Could you check a few things on this drawing? It's one solid part, dimensions in mm from its lowest x, y, z. Give positions to 0.01 mm unless a question says otherwise; leave off trailing zeros. Order: outer loops, then holes, each group sorted by start corner. A loop starts at its lowest first (then second) coordinate and runs counter-clockwise, first axis right, second up. Notation, with made-up numbers: M -14.5,83.25 L 12.5,83.25 A23 ccw 12.5,117.25 Z; hole C 74.25,79.5 d1. An arc over 180 degrees is marked long. Use one line per item in the form item = value.
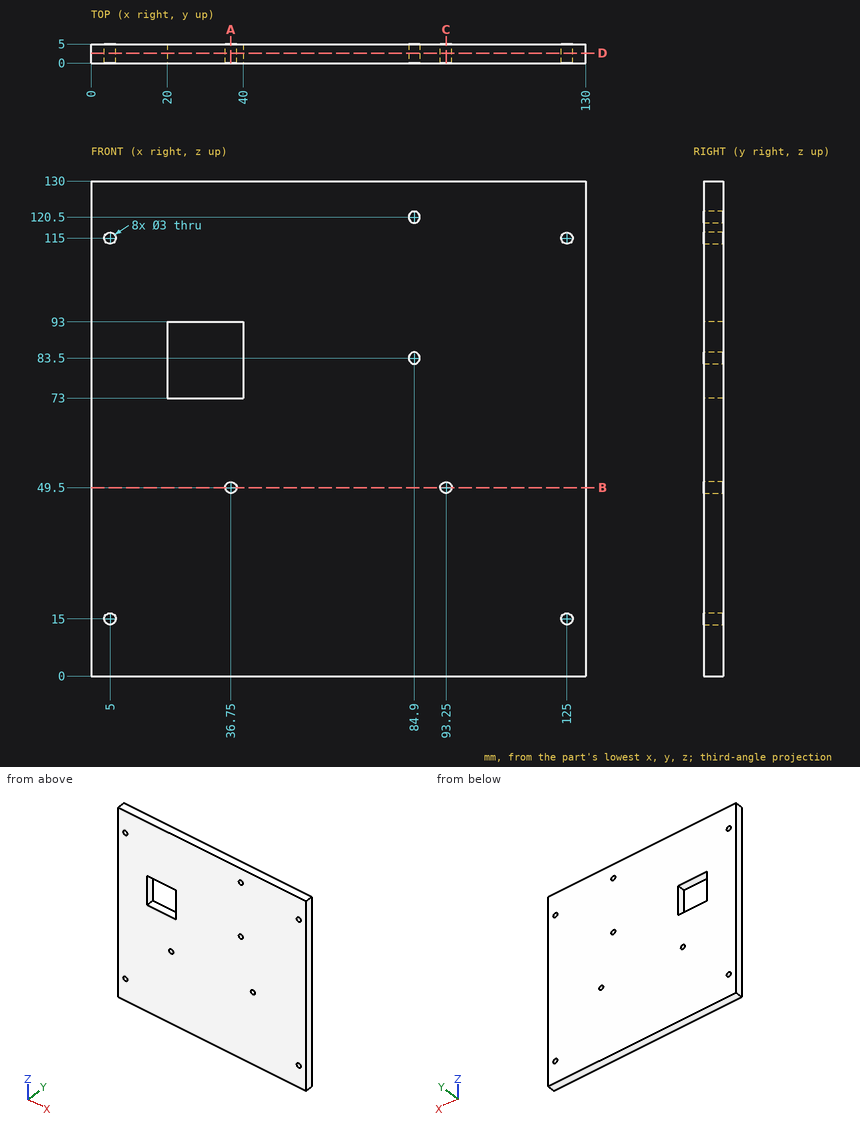
Q1. I want a section at D-D on y = 2.6. State how many separate pieces and enclosed holes the cut face has, then the cut area to 3 significant figures.
Found:
separate_pieces = 1
enclosed_holes = 9
area = 16,400 mm²
Q2. I want a section at B-B on z = 49.5. Write out the boundary of the cut face in (x, y), then the cut area to 3 significant figures.
Found:
outline = M 0,0 L 35.25,0 L 35.25,5 L 0,5 Z; M 38.25,0 L 91.75,0 L 91.75,5 L 38.25,5 Z; M 94.75,0 L 130,0 L 130,5 L 94.75,5 Z
area = 620 mm²
Q3. I want a section at A-A on x = 36.75. Write out the boundary of the cut face in (y, z).
Found:
outline = M 0,0 L 5,0 L 5,48 L 0,48 Z; M 0,51 L 5,51 L 5,73 L 0,73 Z; M 0,93 L 5,93 L 5,130 L 0,130 Z
Q4. I need wall thicknesses on L1, parallel to Z at x = 36.75, y = 1.15; L2, parallel to X at y = 2.8, z = 115; L3, parallel to Z at x = 5, y = 3.05. Which ranges of each line are inside material? Lowest first, please.
Found:
L1 = 0 to 48, 51 to 73, 93 to 130
L2 = 0 to 3.5, 6.5 to 123.5, 126.5 to 130
L3 = 0 to 13.5, 16.5 to 113.5, 116.5 to 130
Q5. I want a section at C-C on x = 93.25. Write out the boundary of the cut face in (y, z).
Found:
outline = M 0,0 L 5,0 L 5,48 L 0,48 Z; M 0,51 L 5,51 L 5,130 L 0,130 Z
Q6. I'm going to push flat-ended pins straight in: pin 1 Ø5 at (x, z) = (74.5, 105) entering from -Y; pin 2 Ø1.8 at (x, z) = (84.9, 120.5) entering from -Y. Where does each tip first touch, or does it pass through?
Found:
pin_1 = 0
pin_2 = through
